Input: part model. Units: mm. Frame: model coordinates. Face numbers are marked on the shaded views. A direction names the side the tool comes from. Coordinates: 2 decimals unless noted, no trailing zeros. Order: outer loops, then holes, each group sorted by start corner. A loop starts at its lowest first (then second) coordinate and runs counter-clockwise, first axis right, second up. Notation, with made-up numbers: (47, 8.5) -> (96, 8.5) arc R19 cw to (96, 13.5) -> close; hole circle Ø3 at (-34.75, -7). An arc over 180 degrees is marked (long way). Use one line per item in the form item = value. Start each with the question number.
1) Access query for the marked faces 1 and 2. Directions: +Z, -Z, +X, -X, +Y, -Y. A direction counts if a zero-diameter tool reaches every point of the face in a straight line with its end or side. Return the directions, or none.
2) Ray query, line 1 along Y through (x, z) = (-28.9, 12.5); line 2 along Z through (x, y) = (-41, -195.5); line 3 along X through (y, z) = (15.5, 23.25). Return the intervals inside material, ascending.
3) Pin query (flat end, axial travel): pin 1 (1 mm diameter, centred on x = -47.5, y = -116.5, fed in from +Z). Return the tip coordinate at first contact, or that it passes through.
4) Section query A-A on z = 12.5. Output: boundary loops of the cut face in (x, y), then the cut area to 3 significant figures.
5) Section query C-C on x = -32. Output: boundary loops of the cut face in (y, z).
6) Section query B-B on y = -83. Output: boundary loops of the cut face in (x, z), then the cut area to 3 significant figures.
from build123d import *

# Parameters (mm, degrees)
CROQUIS1_W              = 24
CROQUIS1_H              = 270
CROQUIS1_R              = 1.5
SALIENTE_EXTRUIR1_DEPTH = 1
CROQUIS2_W              = 1
CROQUIS2_H              = 270
SALIENTE_EXTRUIR2_DEPTH = 25
CROQUIS3_R              = 5
CORTAR_EXTRUIR1_DEPTH   = 1


with BuildPart() as part:
    # Croquis1 → Saliente-Extruir1 (new body)
    with BuildSketch(Plane.XY):
        with Locations((-41.401725042, -108.514805415)):
            Rectangle(CROQUIS1_W, CROQUIS1_H)
        with Locations((-43.401725042, 12.485194585)):
            Circle(CROQUIS1_R, mode=Mode.SUBTRACT)
        with Locations((-43.401725042, -229.514805415)):
            Circle(CROQUIS1_R, mode=Mode.SUBTRACT)
    extrude(amount=SALIENTE_EXTRUIR1_DEPTH)

    # Croquis2 → Saliente-Extruir2 (add)
    with BuildSketch(Plane.XY):
        with Locations((-28.901725042, -108.514805415)):
            Rectangle(CROQUIS2_W, CROQUIS2_H)
    extrude(amount=SALIENTE_EXTRUIR2_DEPTH)

    # Croquis3 → Cortar-Extruir1 (cut)
    with BuildSketch(Plane(origin=(-28.401725042, 0, 0), x_dir=(0, 0, -1), z_dir=(1, 0, 0))):
        with Locations((-12.5, -108.514805415)):
            Circle(CROQUIS3_R)
    extrude(amount=-CORTAR_EXTRUIR1_DEPTH, mode=Mode.SUBTRACT)


solid = part.part
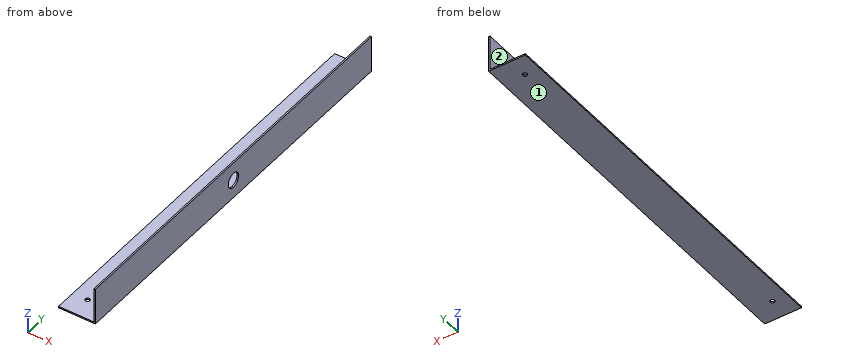
Answers below:
q1.face_1 = -Z, +X, -X, +Y, -Y
q1.face_2 = +Z, -X, +Y, -Y
q2.line_1 = -243.51 to -113.51, -103.51 to 26.49
q2.line_2 = 0 to 1
q2.line_3 = -29.4 to -28.4
q3.pin_1 = 1
q4.outline = (-29.4, -243.51) -> (-28.4, -243.51) -> (-28.4, -113.51) -> (-29.4, -113.51) -> close; (-29.4, -103.51) -> (-28.4, -103.51) -> (-28.4, 26.49) -> (-29.4, 26.49) -> close
q4.area = 260 mm^2
q5.outline = (-243.51, 0) -> (26.49, 0) -> (26.49, 1) -> (-243.51, 1) -> close
q6.outline = (-53.4, 0) -> (-28.4, 0) -> (-28.4, 25) -> (-29.4, 25) -> (-29.4, 1) -> (-53.4, 1) -> close
q6.area = 49.0 mm^2
